Part model, mm, in its own coordinate system. A direction names the side the tool comes from. Give positions to 0.01 mm unless a question says otherwise; leave off trailing zeros. Order: outer loops, then holes, each group sorted by start corner. A loop starts at its lowest first (then second) coordinate and runs counter-clockwise, first axis right, second up. Notation, with made-up numbers: (-23, -1.5) - (13, -1.5) arc R30 cw to (13, 34.5) - close; hole circle Ø5 at (6, -32). An arc over 180 degrees is marked (long way). Use one line per item in the form item = value. Start each with the question number.
1. Band-saw the part on B-B, the plane x = -406. List the corners of the cut face in (y, z).
2. Tool access for faces 4 (the face through (579, -401, -249)), 5 (the face through (-551, -401, -229)), 6 (the face through (539, -401, -249)), 7 (the face through (-571, -401, -249)), 8 (the face through (26.76, 55.39, 51.46)): list every direction of +Z, -Z, +X, -X, +Y, -Y with a clear straight run to the whole face (end or side of a thin tool).
3. Band-saw the part on D-D, the plane x = 370. List the corners of the cut face in (y, z), plus the area to 3 significant figures.
4. Band-saw the part on A-A, the plane y = -515.5. List the corners of the cut face in (x, z), plus the area to 3 significant figures.
5. Pull direction X, two halves, no side cores. Call faces 1 (the face through (-551, -781, -249)), 2 (the face through (539, -401, 251)), 3 (the face through (55.889, 29.487, -17.6)): +X half, -X half, draft (parallel to the pull), parting line (faces both ways), or undercut.
6. Drill centre lines: line 1 (Y direction, x = -537, z = 3.5); line 2 (X direction, y = 10.25, z = 0). Where is each one in solid material? Low to high.
7. Pin check, flat tips, straight feed: P1, Ø12, axis at x = 551, y = -245, coming from the +Z side; P2, Ø12, axis at y = -343.5, z = 256.5, coming from the -X side; P3, Ø10, axis at x = -63.03, z = 0, coming from the -Y side. Stop position of each tip, or through.
8. Band-saw the part on C-C, the plane z = 110. List the corners of the cut face in (x, y).
from build123d import *

# Parameters (mm, degrees)
CORTAR_EXTRUIR1_START   = -50
CROQUIS2_R              = 4.324629937
CORTAR_EXTRUIR1_DEPTH   = 25
CROQUIS3_W              = 1202
CROQUIS3_H              = 602
SALIENTE_EXTRUIR1_DEPTH = 31
CROQUIS4_W              = 40
CROQUIS4_H              = 40
SALIENTE_EXTRUIR2_DEPTH = 750
CROQUIS5_W              = 210.655681701
CROQUIS5_H              = 149.539527133
SALIENTE_EXTRUIR3_DEPTH = 70


with BuildPart() as part:
    # Croquis1 → Revolución1 (revolve)
    with BuildSketch(Plane.XY, mode=Mode.PRIVATE) as revoluci_n1_sk:
        Polygon((0, 0), (0, 80), (-58, 80), (-58, 31.455108359), (-67.5, 0), align=None)
    revolve(revoluci_n1_sk.sketch.rotate(Axis((0, 0, 0), (0, 1, 0)), 180), axis=Axis((0, 0, 0), (0, 1, 0)))

    # Croquis2 → Cortar-Extruir1 (cut)
    with BuildSketch(Plane(origin=(0, 80, 0), x_dir=(1, 0, 0), z_dir=(0, 1, 0)).offset(CORTAR_EXTRUIR1_START)):
        with Locations((0, 63.025248345)):
            Circle(CROQUIS2_R)
        with Locations((63.025248345, 0)):
            Circle(CROQUIS2_R)
        with Locations((0, -63.025248345)):
            Circle(CROQUIS2_R)
        with Locations((-63.025248345, 0)):
            Circle(CROQUIS2_R)
    extrude(amount=-CORTAR_EXTRUIR1_DEPTH, mode=Mode.SUBTRACT)

    # Croquis3 → Saliente-Extruir1 (add)
    with BuildSketch(Plane.XZ):
        Rectangle(CROQUIS3_W, CROQUIS3_H)
    extrude(amount=SALIENTE_EXTRUIR1_DEPTH)

    # Croquis4 → Saliente-Extruir2 (add)
    with BuildSketch(Plane.XZ.offset(31)):
        with Locations((-551, 251)):
            Rectangle(CROQUIS4_W, CROQUIS4_H)
        with Locations((559, 251)):
            Rectangle(CROQUIS4_W, CROQUIS4_H)
        with Locations((559, -249)):
            Rectangle(CROQUIS4_W, CROQUIS4_H)
        with Locations((-551, -249)):
            Rectangle(CROQUIS4_W, CROQUIS4_H)
    extrude(amount=SALIENTE_EXTRUIR2_DEPTH)

    # Croquis5 → Saliente-Extruir3 (add)
    with BuildSketch(Plane(origin=(0, 0, 0), x_dir=(1, 0, 0), z_dir=(0, 1, 0))):
        with Locations((-484.76769938, -216.371921998)):
            Rectangle(CROQUIS5_W, CROQUIS5_H)
    extrude(amount=SALIENTE_EXTRUIR3_DEPTH)


solid = part.part
From the geometry:
q1.outline = (-31, -301) - (0, -301) - (0, 141.6) - (70, 141.6) - (70, 291.14) - (0, 291.14) - (0, 301) - (-31, 301) - close
q2.face_4 = +Z, -Z, +X, -Y
q2.face_5 = +X, -X, -Y
q2.face_6 = +Z, -Z, -Y
q2.face_7 = +Z, -Z, -X, -Y
q2.face_8 = +Y
q3.outline = (-31, -301) - (0, -301) - (0, 301) - (-31, 301) - close
q3.area = 18,700 mm²
q4.outline = (-571, -269) - (-531, -269) - (-531, -229) - (-571, -229) - close; (-571, 231) - (-531, 231) - (-531, 271) - (-571, 271) - close; (539, -269) - (579, -269) - (579, -229) - (539, -229) - close; (539, 231) - (579, 231) - (579, 271) - (539, 271) - close
q4.area = 6,400 mm²
q5.face_1 = draft
q5.face_2 = undercut
q5.face_3 = parting line
q6.line_1 = -31 to 0
q6.line_2 = -58.7 to 58.7
q7.P1 = 271
q7.P2 = -571
q7.P3 = -31
q8.outline = (-601, -31) - (601, -31) - (601, 0) - (-601, 0) - close
